Design review of the part built by this model. Coordinates are the model's own, in mm. Face numbers are marked on the shaded views. A direction names the side the tool comes from. Give positions to 0.01 mm unless a question says otherwise; leave off trailing zeros. Loops run counter-clockwise (first coordinate to the right, second up) from the corner with the lowest first, then second, coordinate; pieces in that order, holes last.
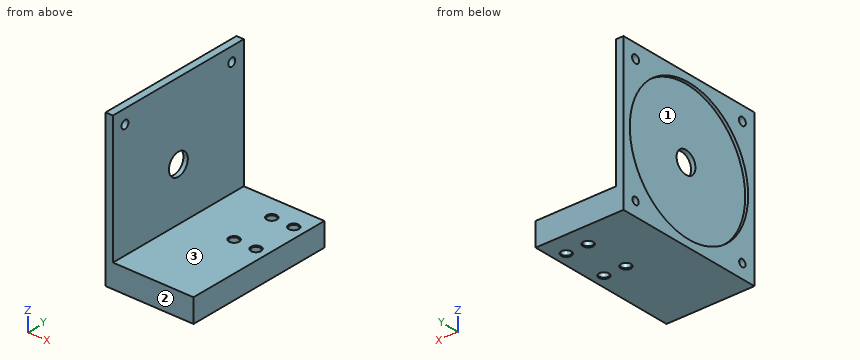
from build123d import *

# Parameters (mm, degrees)
F0_W      = 104
F0_H      = 104
F1_DEPTH  = 5
F2_R      = 2.75
F3_DEPTH  = 5.001
F4_W      = 104
F4_H      = 16
F5_DEPTH  = 55
F6_R      = 2.5
F7_DEPTH  = 12
F9_R      = 47
F10_DEPTH = 2
F11_R     = 7.5
F12_DEPTH = 58.001
F8_R      = 3
F13_DEPTH = 16.001
F14_SIZE  = 0.5


with BuildPart() as f1:
    # F0 (on Right) → F1 (new body)
    with BuildSketch(Plane.YZ):
        Rectangle(F0_W, F0_H)
    extrude(amount=F1_DEPTH)

    # F2 (on face) → F3 (cut, through all)
    with BuildSketch(Plane.YZ.offset(5)):
        with Locations((42.426407, 42.426407)):
            Circle(F2_R)
        with Locations((-42.426407, 42.426407)):
            Circle(F2_R)
    extrude(amount=-F3_DEPTH, mode=Mode.SUBTRACT)

    # F4 (on face) → F5 (join)
    with BuildSketch(Plane.YZ.offset(5)):
        with Locations((0, -44)):
            Rectangle(F4_W, F4_H)
    extrude(amount=F5_DEPTH)

    # F6 (on face) → F7 (cut)
    with BuildSketch(Plane(origin=(0, 0, 0), x_dir=(0, -1, 0), z_dir=(-1, 0, 0))):
        with Locations((-42.426407, -42.426407)):
            Circle(F6_R)
        with Locations((42.426407, -42.426407)):
            Circle(F6_R)
    extrude(amount=-F7_DEPTH, mode=Mode.SUBTRACT)

    # F9 (on face) → F10 (cut)
    with BuildSketch(Plane(origin=(0, 0, 0), x_dir=(0, -1, 0), z_dir=(-1, 0, 0))):
        Circle(F9_R)
    extrude(amount=-F10_DEPTH, mode=Mode.SUBTRACT)

    # F11 (on face) → F12 (cut, through all)
    with BuildSketch(Plane(origin=(2, 0, 0), x_dir=(0, -1, 0), z_dir=(-1, 0, 0))):
        Circle(F11_R)
    extrude(amount=-F12_DEPTH, mode=Mode.SUBTRACT)

    # F8 (on face) → F13 (cut, through all)
    with BuildSketch(Plane.XY.offset(-36)):
        with Locations((52, 37)):
            Circle(F8_R)
        with Locations((52, 7)):
            Circle(F8_R)
        with Locations((37, 37)):
            Circle(F8_R)
        with Locations((37, 7)):
            Circle(F8_R)
    extrude(amount=-F13_DEPTH, mode=Mode.SUBTRACT)

    # F14
    f14_edges = [f1.edges().sort_by_distance(p)[0] for p in [
        (34, 37, -36),
        (40, 37, -44),
        (34, 37, -52),
        (49, 37, -36),
        (55, 37, -44),
        (49, 37, -52),
        (34, 7, -36),
        (40, 7, -44),
        (34, 7, -52),
        (49, 7, -36),
        (55, 7, -44),
        (49, 7, -52),
    ]]
    chamfer(f14_edges, length=F14_SIZE)


solid = f1.part
Q1. Take a section at C-C (z = 0). Give the boundary of the cut face in (x, y).
Results:
outline: (0, -52) - (5, -52) - (5, -7.5) - (2, -7.5) - (2, -47) - (0, -47) - close; (0, 47) - (2, 47) - (2, 7.5) - (5, 7.5) - (5, 52) - (0, 52) - close
Q2. Wall thickness on line 1 (Z direction, x = 3.7, y = 0); line 2 (Z direction, x = 34, y = 21.5); line 3 (Y direction, x = 53, z = -38): over which ranges is each line inside the solid? List them lowest first.
Results:
line 1: z = -52 to -7.5, 7.5 to 52
line 2: z = -52 to -36
line 3: y = -52 to 4.17, 9.83 to 34.17, 39.83 to 52
Q3. Take a section at B-B (y = 0). Give the boundary of the cut face in (x, z), plus the area to 3 significant figures.
Results:
outline: (0, -52) - (60, -52) - (60, -36) - (5, -36) - (5, -7.5) - (2, -7.5) - (2, -47) - (0, -47) - close; (0, 47) - (2, 47) - (2, 7.5) - (5, 7.5) - (5, 52) - (0, 52) - close
area: 1,170 mm2
Q4. Insertion check: pin 1 (16.5 mm diameter, centred on x = 40, y = 21, fed in from +Z); pin 2 (5.5 mm diameter, centred on y = 43.5, z = -42, fed in from -X); pin 3 (12 mm diameter, centred on y = -30.5, z = -17.5, fed in from +X); pin 4 (3 mm diameter, centred on y = 42.43, z = -42.43, fed in from -X). Each pin has a flat end and moves straight along its axis. Give the tip position at first contact, or say it passes through.
Results:
pin 1: stops at z = -36
pin 2: stops at x = 0
pin 3: stops at x = 5
pin 4: stops at x = 12
Q5. Tool access review of the marked faces 1, 2 and 3: name each direction out of +Z, -Z, +X, -X, +Y, -Y from which nothing blocks a thin tool from reaching the whole face with its end or side.
Results:
face 1: -X
face 2: +Z, -Z, +X, -X, -Y
face 3: +Z, +X, +Y, -Y
Q6. Take a section at A-A (x = 37). Give the boundary of the cut face in (y, z).
Results:
outline: (-52, -52) - (3.5, -52) - (4, -51.5) - (4, -36.5) - (3.5, -36) - (-52, -36) - close; (10, -51.5) - (10.5, -52) - (33.5, -52) - (34, -51.5) - (34, -36.5) - (33.5, -36) - (10.5, -36) - (10, -36.5) - close; (40, -51.5) - (40.5, -52) - (52, -52) - (52, -36) - (40.5, -36) - (40, -36.5) - close
Q7. Take a section at D-D (y = 37). Give the boundary of the cut face in (x, z), plus the area to 3 significant figures.
Results:
outline: (0, -52) - (33.5, -52) - (34, -51.5) - (34, -36.5) - (33.5, -36) - (5, -36) - (5, 52) - (0, 52) - (0, 28.98) - (2, 28.98) - (2, -28.98) - (0, -28.98) - close; (40, -51.5) - (40.5, -52) - (48.5, -52) - (49, -51.5) - (49, -36.5) - (48.5, -36) - (40.5, -36) - (40, -36.5) - close; (55, -51.5) - (55.5, -52) - (60, -52) - (60, -36) - (55.5, -36) - (55, -36.5) - close
area: 1,090 mm2
